Study the drawing (mm; zero at the part's minimum x, y, z) and answer. A direction names the side the tool comes from. Coordinates: 2 decimals unless noted, no trailing zeros. Loops run counter-clockwise (first coordinate to the right, second up) from the corner with the lowest first, then second, coordinate; pieces in that order, holes last. Notation, with made-up numbers: (31.5, 55) -> (72.5, 55) arc R7 cw to (72.5, 64) -> close; hole circle Ø3 at (-21, -15.5). An arc over 180 degrees is marked (long way). Answer as CSV lines item,"result".
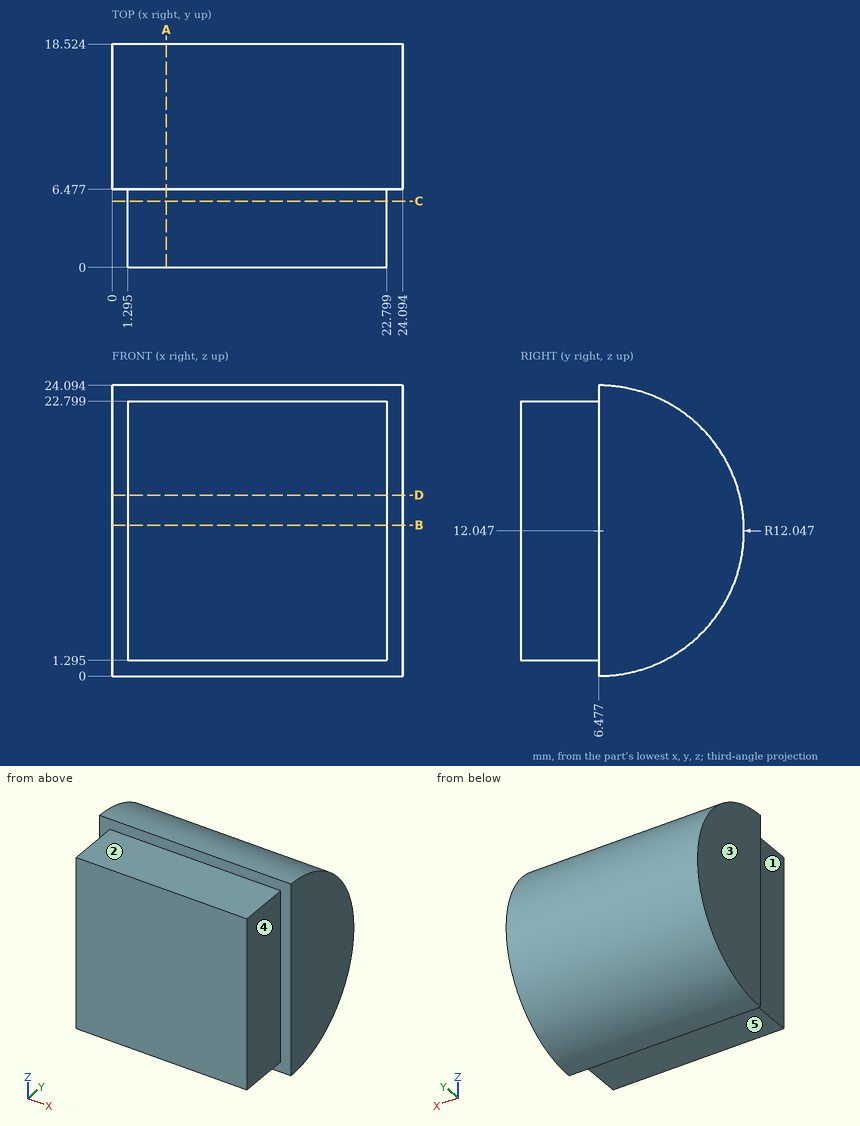
Q1. Given pin 1 Ø8 at (x, z) = (18, 21.5) entering from +Y; pin 2 Ø5 at (y, z) = (3.5, 10.5) entering from +X; pin 3 Ø1.9 at (y, z) = (4.5, 11.5) entering from -X (1 decimal), each flat-ended and moving along its own axis, determine where each tip first touches the part or whether it passes through.
Results:
pin 1,"stops at y = 17.22"
pin 2,"stops at x = 22.8"
pin 3,"stops at x = 1.3"
Q2. A cutting plane is placed at A-A, the plane x = 4.5. Write down the section's boundary in (y, z) (1 decimal), and give its area (3 significant figures).
Results:
outline,"(0, 1.3) -> (6.5, 1.3) -> (6.5, 0) arc R12 ccw to (6.5, 24.1) -> (6.5, 22.8) -> (0, 22.8) -> close"
area,"367 mm²"
Q3. A cutting plane is placed at D-D, the plane z = 15. Write down the section's boundary in (x, y) (1 decimal), and give its area (3 significant figures).
Results:
outline,"(0, 6.5) -> (1.3, 6.5) -> (1.3, 0) -> (22.8, 0) -> (22.8, 6.5) -> (24.1, 6.5) -> (24.1, 18.2) -> (0, 18.2) -> close"
area,"421 mm²"
Q4. A cutting plane is placed at B-B, the plane z = 12.5. Write down the section's boundary in (x, y) (1 decimal), and give its area (3 significant figures).
Results:
outline,"(0, 6.5) -> (1.3, 6.5) -> (1.3, 0) -> (22.8, 0) -> (22.8, 6.5) -> (24.1, 6.5) -> (24.1, 18.5) -> (0, 18.5) -> close"
area,"429 mm²"
Q5. A cutting plane is placed at C-C, the plane y = 5.5. Write down the section's boundary in (x, z) (1 decimal), and give its area (3 significant figures).
Results:
outline,"(1.3, 1.3) -> (22.8, 1.3) -> (22.8, 22.8) -> (1.3, 22.8) -> close"
area,"462 mm²"
Q6. Find the intervals of material crossed by probe 1 along X at (y, z) = (1.5, 13.5) (1 decimal); probe 2 along Y at (x, z) = (16.25, 12.25), in increasing order. Write a range as [from, to].
Results:
probe 1,"x = [1.3, 22.8]"
probe 2,"y = [0, 18.52]"
Q7. For the marked faces 1, 2, 3, 4 and 5, determine the directions among +Z, -Z, +X, -X, +Y, -Y from which every point of the face is accessible in a straight line to the end or side of a thin tool.
Results:
face 1,"+Z, -Z, -X, -Y"
face 2,"+Z, +X, -X, -Y"
face 3,"+Z, -Z, -X, +Y, -Y"
face 4,"+Z, -Z, +X, -Y"
face 5,"-Z, +X, -X, -Y"
